Autodesk Inventor part; units mm, degrees
ref_plane "YZ Plane" through (0, 0, 0) normal (1, 0, 0) x (0, 1, 0)
ref_plane "XZ Plane" through (0, 0, 0) normal (0, 1, 0) x (-1, 0, 0)
ref_plane "XY Plane" through (0, 0, 0) normal (0, 0, 1) x (1, 0, 0)
sketch "Sketch1" plane through (0, 0, 0) normal (0, 1, 0) x (-1, 0, 0)
  line L0 (-6.1, 4.9) -> (6.1, 4.9)
  line L1 (6.1, 4.9) -> (6.1, -4.9)
  line L2 (6.1, -4.9) -> (-6.1, -4.9)
  line L3 (-6.1, -4.9) -> (-6.1, 4.9)
  line L4 (-6.1, 4.9) -> (6.1, -4.9) construction
  line L5 (6.1, 4.9) -> (-6.1, -4.9) construction
  point P0 (0, 0)
  dimension "d0" = 12.2
  dimension "d1" = 9.8
extrude "Extrusion1" add sketch "Sketch1" along normal blind 5.1
sketch "Sketch2" plane through (6.1, 0, 4.9) normal (1, 0, 0) x (0, 0, -1)
  line L0 (4.9, 0) -> (4.9, 2.55)
  line L1 (0, 0) -> (0, 5.1)
  line L2 (8.9, 1.55) -> (0.9, 1.55)
  line L3 (0.9, 1.55) -> (0.9, 3.55)
  line L4 (0.9, 3.55) -> (8.9, 3.55)
  line L5 (8.9, 3.55) -> (8.9, 1.55)
  line L6 (8.9, 1.55) -> (0.9, 3.55) construction
  line L7 (0.9, 1.55) -> (8.9, 3.55) construction
  dimension "d4" = 2.55
  dimension "d5" = 8
  dimension "d6" = 2
extrude "Extrusion2" cut sketch "Sketch2" against normal up to next
sketch "Sketch3" plane through (6.1, 1.55, 4) normal (0, 1, 0) x (1, 0, 0)
  line L0 (-12.2, 8.9) -> (-12.2, -0.9)
  line L1 (-12.2, 4) -> (-9.2, 4)
  line L2 (0, 0) -> (0, 8)
  line L3 (0, 4) -> (-3, 4)
  circle A0 centre (-3, 4) radius 3
  circle A1 centre (-9.2, 4) radius 3
  point P0 (-6.1, 4)
  dimension "d9" = 3
  dimension "d10" = 3
  dimension "d11" = 6
  dimension "d12" = 6
extrude "Extrusion3" add sketch "Sketch3" along normal up to next
sketch "Sketch4" plane through (0, 0, 0) normal (0, -1, 0) x (1, 0, 0)
  line L0 (6.1, 4.9) -> (-6.1, 4.9)
  line L1 (0, 4.9) -> (0, 4.25)
  line L2 (1.1, 3.6) -> (-1.1, 3.6)
  line L3 (-1.1, 3.6) -> (-1.1, 4.9)
  line L4 (-1.1, 4.9) -> (1.1, 4.9)
  line L5 (1.1, 4.9) -> (1.1, 3.6)
  line L6 (1.1, 3.6) -> (-1.1, 4.9) construction
  line L7 (-1.1, 3.6) -> (1.1, 4.9) construction
  line L8 (6.1, -4.9) -> (-6.1, -4.9)
  line L9 (-6.1, -4.9) -> (-4.75, -4.9)
  line L10 (-4.75, -4.9) -> (-3.65, -4.9)
  line L11 (-3.65, -4.9) -> (-3.65, -3.9)
  line L12 (-3.65, -4.9) -> (-2.65, -4.9) construction
  line L13 (-2.55, -2.9) -> (-4.75, -2.9)
  line L14 (-4.75, -2.9) -> (-4.75, -4.9)
  line L15 (-4.75, -4.9) -> (-2.55, -4.9)
  line L16 (-2.55, -4.9) -> (-2.55, -2.9)
  line L17 (-2.55, -2.9) -> (-4.75, -4.9) construction
  line L18 (-4.75, -2.9) -> (-2.55, -4.9) construction
  line L19 (4.75, -2.9) -> (2.55, -2.9)
  line L20 (4.75, -4.9) -> (4.75, -2.9)
  line L21 (3.65, -4.9) -> (4.65, -4.9) construction
  line L22 (2.55, -2.9) -> (2.55, -4.9)
  line L23 (2.55, -4.9) -> (4.75, -4.9)
  point P0 (0, 0)
  dimension "d15" = 0.65
  dimension "d16" = 2.2
  dimension "d17" = 1.3
  dimension "d18" = 1.35
  dimension "d19" = 1.1
  dimension "d20" = 1
  dimension "d21" = 90
  dimension "d22" = 2.2
  dimension "d23" = 2
  dimension "d26" = 7.3
extrude "Extrusion4" add sketch "Sketch4" along normal blind 0.3
sketch "Sketch5" plane through (0, 5.1, 0) normal (0, 1, 0) x (1, 0, 0)
  line L0 (6.1, 4.9) -> (-6.1, 4.9)
  line L1 (-6.1, 4.9) -> (-3.65, 4.9)
  line L2 (-3.65, 4.9) -> (-3.65, 3.9)
  circle A0 centre (-3.65, 3.9) radius 0.5
  point P0 (0, 0)
  dimension "d33" = 2.45
  dimension "d34" = 1
  dimension "d35" = 1
extrude "Extrusion5" add sketch "Sketch5" along normal blind 0.1
sketch "Sketch6" plane through (0, 5.1, 0) normal (0, 1, 0) x (1, 0, 0)
  line L0 (-4.0529, 1.1605) -> (0.3424, 1.1605) construction
  line L1 (0.3424, 1.1605) -> (0.3424, 0.2782) construction
  line L2 (0.3424, 0.2782) -> (-4.0529, 0.2782) construction
  line L3 (-4.0529, 0.2782) -> (-4.0529, 1.1605) construction
  point P0 (0, 0)
  dimension "d1" = 9.8
properties part number "HCV1206"
Work out the finished part from the listing and answer in its coordinate system (mm). A direction names the side the tool comes from. Round coordinates to 2 decimals unless told otherwise and drop trailing zeros. Loops run counter-clockwise (first coordinate to the right, second up) from the corner with the lowest first, then second, coordinate; pieces in that order, holes last. Notation, with made-up numbers: (-39, -20.75) - (14, -20.75) arc R26 cw to (14, 10.25) - close; hole circle Ø2 at (-24, -33). An arc over 180 degrees is marked (long way). One line per item, written item: value.
Q1. Find section D-D on x = 1.5. Give the vertices of the cut face in (y, z), and give its area (3 significant figures).
Check values:
outline: (0, -4.9) - (5.1, -4.9) - (5.1, 4.9) - (0, 4.9) - close; hole (1.55, -4) - (3.55, -4) - (3.55, -2.54) - (1.55, -2.54) - close; hole (1.55, 2.54) - (3.55, 2.54) - (3.55, 4) - (1.55, 4) - close
area: 44.1 mm2
Q2. For faces 1 (the flat face through (0, 3, 4)), 2 (the flat face through (0, 3.55, 1)), 3 (the flat face through (4, -0.3, -4)), determine the directions among +Z, -Z, +X, -X, +Y, -Y from which every point of the face is accessible in a straight line to the end or side of a thin tool.
Check values:
face 1: +X, -X
face 2: none
face 3: +Z, -Z, +X, -X, -Y
Q3. Find section C-C on z = -1.5. Give the vertices of the cut face in (x, y), and give its area (3 significant figures).
Check values:
outline: (-6.1, 0) - (6.1, 0) - (6.1, 1.55) - (5.7, 1.55) - (5.7, 3.55) - (6.1, 3.55) - (6.1, 5.1) - (-6.1, 5.1) - (-6.1, 3.55) - (-5.7, 3.55) - (-5.7, 1.55) - (-6.1, 1.55) - close; hole (-0.5, 1.55) - (0.5, 1.55) - (0.5, 3.55) - (-0.5, 3.55) - close
area: 58.6 mm2
Q4. Straight lines are drawn through the part: probe 1 along Z at (x, y) = (-2, 2.75); probe 2 along Y at (x, z) = (3, 3.75); probe 3 along Z at (x, y) = (-3.75, 2.7). For each, find the intervals that lie inside material, in ascending order.
Check values:
probe 1: -4.9 to -4, -2.79 to 2.79, 4 to 4.9
probe 2: 0 to 1.55, 3.55 to 5.1
probe 3: -4.9 to -4, -2.93 to 2.93, 4 to 4.9
Q5. The mould has two halves that part along Z. Classify faces 4 (the flat face through (-4, -0.3, -4)), 5 (the flat face through (0, 3, -4)), 6 (the flat face through (0, 2, 4.9)): +Z half, -Z half, draft (parallel to the pull), parting line (faces both ways), or undercut.
Check values:
face 4: draft
face 5: undercut
face 6: +Z half
Q6. Find section A-A on y = 2.85. Give the vertices of the cut face in (x, z).
Check values:
outline: (-6.1, -4.9) - (6.1, -4.9) - (6.1, -4) - (-6.1, -4) - close; circle Ø6 at (-3.1, 0); (-6.1, 4) - (6.1, 4) - (6.1, 4.9) - (-6.1, 4.9) - close; circle Ø6 at (3.1, 0)
Q7. Each of these flat-tipped pins is pushed along its axis until it touches: pin 1 Ø3 at (x, z) = (-1.5, -2) entering from -Y; pin 2 Ø4 at (x, z) = (-4, 2) entering from -Y. Where does it stop, or does it pass through?
Check values:
pin 1: y = -0.3
pin 2: y = 0
Q8. Find section B-B on x = -3.65. Give the vertices of the cut face in (y, z), and give its area (3 significant figures).
Check values:
outline: (-0.3, -4.9) - (5.1, -4.9) - (5.1, -4.4) - (5.2, -4.4) - (5.2, -3.4) - (5.1, -3.4) - (5.1, 4.9) - (0, 4.9) - (0, -2.9) - (-0.3, -2.9) - close; hole (1.55, -4) - (3.55, -4) - (3.55, -2.95) - (1.55, -2.95) - close; hole (1.55, 2.95) - (3.55, 2.95) - (3.55, 4) - (1.55, 4) - close
area: 46.5 mm2
